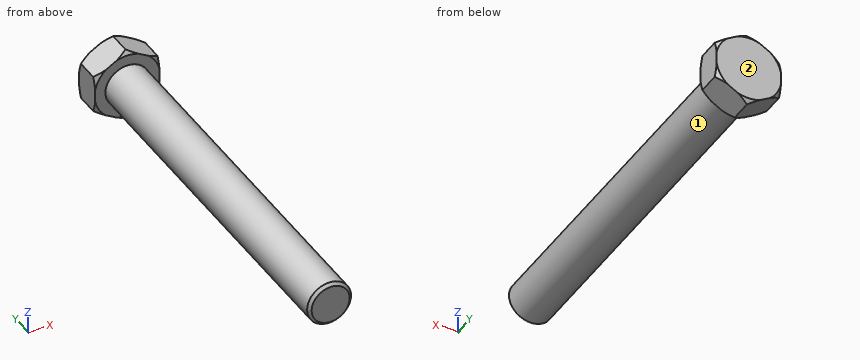
```python
from build123d import *

# Parameters (mm, degrees)
BOSS_EXTRUDE1_DEPTH = 10
SKETCH2_R           = 7.5
BOSS_EXTRUDE2_DEPTH = 126
CHAMFER1_SIZE       = 1
SCALE1_SCALE        = 0.18
SCALE2_SCALE        = 1.04


with BuildPart() as part:
    # Sketch1 → Boss-Extrude1 (new body)
    with BuildSketch(Plane(origin=(0, 0, 0), x_dir=(1, 0, 0), z_dir=(0, 1, 0))):
        Polygon((0, 12.701705922), (-11, 6.350852961), (-11, -6.350852961), (0, -12.701705922), (11, -6.350852961), (11, 6.350852961), align=None)
    extrude(amount=BOSS_EXTRUDE1_DEPTH)

    # Sketch2 → Boss-Extrude2 (add)
    with BuildSketch(Plane.XZ):
        Circle(SKETCH2_R)
    extrude(amount=BOSS_EXTRUDE2_DEPTH)

    # Chamfer1
    chamfer1_edges = [part.edges().sort_by_distance(p)[0] for p in [
        (-7.5, -126, 0),
    ]]
    chamfer(chamfer1_edges, length=CHAMFER1_SIZE)

    # Sketch4 → Cut-Revolve2 (revolve, cut)
    with BuildSketch(Plane(origin=(0, 0, 0), x_dir=(0, 0, -1), z_dir=(1, 0, 0))):
        Polygon((-12.701705922, 10), (-12.701705922, 8.8), (-11.201705922, 10), align=None)
        Polygon((-12.701705922, 0), (-12.701705922, 1.2), (-11.201705922, 0), align=None)
    revolve(axis=Axis((0, 0, 0), (0, 1, 0)), mode=Mode.SUBTRACT)


with BuildPart() as part_1:
    # Scale1: scaled about (0, -52.210522466, 0)
    add(part.part.scale(SCALE1_SCALE).moved(Location((0, -42.812628422, 0))))


with BuildPart() as part_2:
    # Scale2: scaled about (0, -52.210522466, 0)
    add(part_1.part.scale(SCALE2_SCALE).moved(Location((0, 2.088420899, 0))))


solid = part_2.part
```
Geometry check sheet. Reference: the model listing, model coordinates, mm. Face numbers are marked on the shaded views. A direction names the side the tool comes from. Round coordinates to 2 decimals unless told otherwise and drop trailing zeros. Loops run counter-clockwise (first coordinate to the right, second up) from the corner with the lowest first, then second, coordinate; pieces in that order, holes last. Notation, with made-up numbers: (-34.5, 9) - (7.5, 9) arc R23 cw to (7.5, 32) - close; hole circle Ø6 at (14, 5.5). An arc over 180 degrees is marked (long way). Use a Markdown table: item, result.
Q1. Access from +Z, -Z, +X, -X, +Y, -Y to the whole of each face (thin tool, end or side, straight path). Record for the marked faces 1 and 2.
Solutions:
| item | result |
|---|---|
| face 1 | -Y |
| face 2 | +Z, -Z, +X, -X, +Y |
Q2. Material ranges on line 1 (X direction, y = -58.75, z = 0.75); line 2 (Y direction, x = -1.35, z = 1.05); line 3 (Z direction, x = 0.1, y = -58.75), recorded low to high.
Solutions:
| item | result |
|---|---|
| line 1 | x = -1.19 to 1.19 |
| line 2 | y = -42.44 to -40.56 |
| line 3 | z = -1.4 to 1.4 |
Q3. Go/stop test with flat-tipped pins: P1, Ø2, axis at y = -60, z = 1.5, coming from the +X side; P2, Ø1, axis at x = -1, y = -54, coming from the -Z side. Record where each tip stops, or that it passes through.
Solutions:
| item | result |
|---|---|
| P1 | stops at x = 1.31 |
| P2 | stops at z = -1.31 |
Q4. Cross-section at A-A on z = 0. Record the cut outline in (x, y), plus the area to 3 significant figures.
Solutions:
| item | result |
|---|---|
| outline | (-2.06, -42.44) - (-1.4, -42.44) - (-1.4, -65.84) - (-1.22, -66.02) - (1.22, -66.02) - (1.4, -65.84) - (1.4, -42.44) - (2.06, -42.44) - (2.06, -40.56) - (-2.06, -40.56) - close |
| area | 73.9 mm2 |
Q5. Cross-section at B-B on y = -51.5. Record the cut outline in (x, z).
Solutions:
| item | result |
|---|---|
| outline | circle Ø2.81 at (0, 0) |
